Source: CAD feature listing. Evaluate the final solid. Frame: model axes, mm. Face numbers are marked on the shaded views. A direction names the side the tool comes from. Give positions to 0.01 mm unless a question says otherwise; leave off trailing zeros. Write each loop counter-clockwise with the first axis right and the second up, starting at its lowest first coordinate (ties: lowest second). Pieces come first, ordered by that corner, then holes. Notation, with made-up numbers: (18, 88.5) - (58, 88.5) arc R22 ccw to (58, 113.5) - close; hole circle Ø11 at (9, -25.5). An arc over 180 degrees is marked (long way). Answer as a JSON object with one key per item and string values. Group by question number.
from build123d import *

# Parameters (mm, degrees)
SKETCH1_R           = 2.794
BOSS_EXTRUDE1_DEPTH = 12.7
SKETCH2_R           = 1.778
CUT_EXTRUDE1_DEPTH  = 49.178879085
SKETCH4_R           = 4.953
CUT_EXTRUDE3_DEPTH  = 3.302
FILLET1_R           = 2.54
CUT_EXTRUDE4_DEPTH  = 3.302


with BuildPart() as part:
    # Sketch1 → Boss-Extrude1 (new body)
    with BuildSketch(Plane.XY):
        with BuildLine():
            ThreePointArc((28.575, 29.21), (27.831051224, 31.006051224), (26.035, 31.75))
            Line((26.035, 31.75), (16.32506331, 31.75))
            ThreePointArc((16.32506331, 31.75), (9.9441, 36.6522), (3.56313669, 31.75))
            Line((3.56313669, 31.75), (-3.56313669, 31.75))
            ThreePointArc((-3.56313669, 31.75), (-9.9441, 36.6522), (-16.32506331, 31.75))
            Line((-16.32506331, 31.75), (-26.035, 31.75))
            ThreePointArc((-26.035, 31.75), (-27.831051224, 31.006051224), (-28.575, 29.21))
            Line((-28.575, 29.21), (-28.575, -29.21))
            ThreePointArc((-28.575, -29.21), (-27.831051224, -31.006051224), (-26.035, -31.75))
            Line((-26.035, -31.75), (-16.32506331, -31.75))
            ThreePointArc((-16.32506331, -31.75), (-9.9441, -36.6522), (-3.56313669, -31.75))
            Line((-3.56313669, -31.75), (3.56313669, -31.75))
            ThreePointArc((3.56313669, -31.75), (9.9441, -36.6522), (16.32506331, -31.75))
            Line((16.32506331, -31.75), (26.035, -31.75))
            ThreePointArc((26.035, -31.75), (27.831051224, -31.006051224), (28.575, -29.21))
            Line((28.575, -29.21), (28.575, 29.21))
        make_face()
        with Locations((-9.9441, 30.0482)):
            Circle(SKETCH1_R, mode=Mode.SUBTRACT)
        with Locations((9.9441, 30.0482)):
            Circle(SKETCH1_R, mode=Mode.SUBTRACT)
        with Locations((9.9441, -30.0482)):
            Circle(SKETCH1_R, mode=Mode.SUBTRACT)
        with Locations((-9.9441, -30.0482)):
            Circle(SKETCH1_R, mode=Mode.SUBTRACT)
    extrude(amount=BOSS_EXTRUDE1_DEPTH)

    # Sketch2 → Cut-Extrude1 (cut, through all)
    with BuildSketch(Plane.XY.offset(12.7)):
        with Locations((-22.098, 19.3675)):
            Circle(SKETCH2_R)
        with Locations((-22.098, -12.5095)):
            Circle(SKETCH2_R)
        with Locations((22.606, -8.3693)):
            Circle(SKETCH2_R)
    extrude(amount=-CUT_EXTRUDE1_DEPTH, mode=Mode.SUBTRACT)

    # Sketch4 → Cut-Extrude3 (cut)
    with BuildSketch(Plane.XY.offset(12.7)):
        with Locations((-9.9441, 30.0482)):
            Circle(SKETCH4_R)
        with Locations((9.9441, 30.0482)):
            Circle(SKETCH4_R)
        with Locations((-9.9441, -30.0482)):
            Circle(SKETCH4_R)
        with Locations((9.9441, -30.0482)):
            Circle(SKETCH4_R)
    extrude(amount=-CUT_EXTRUDE3_DEPTH, mode=Mode.SUBTRACT)

    # Fillet1
    fillet1_edges = [part.edges().sort_by_distance(p)[0] for p in [
        (16.32506331, 31.75, 6.35),
        (16.32506331, -31.75, 6.35),
        (3.56313669, -31.75, 6.35),
        (-3.56313669, -31.75, 6.35),
        (-16.32506331, -31.75, 6.35),
        (-16.32506331, 31.75, 6.35),
        (-3.56313669, 31.75, 6.35),
        (3.56313669, 31.75, 6.35),
    ]]
    fillet(fillet1_edges, radius=FILLET1_R)

    # Sketch3 → Cut-Extrude4 (cut)
    with BuildSketch(Plane(origin=(0, 0, 0), x_dir=(-1, 0, 0), z_dir=(0, 0, -1))):
        Polygon((-22.606, -12.475415114), (-19.05, -10.422357557), (-19.05, -6.316242443), (-22.606, -4.263184886), (-26.162, -6.316242443), (-26.162, -10.422357557), align=None)
        Polygon((22.098, -16.615615114), (25.654, -14.562557557), (25.654, -10.456442443), (22.098, -8.403384886), (18.542, -10.456442443), (18.542, -14.562557557), align=None)
        Polygon((22.098, 15.261384886), (25.654, 17.314442443), (25.654, 21.420557557), (22.098, 23.473615114), (18.542, 21.420557557), (18.542, 17.314442443), align=None)
    extrude(amount=-CUT_EXTRUDE4_DEPTH, mode=Mode.SUBTRACT)


solid = part.part
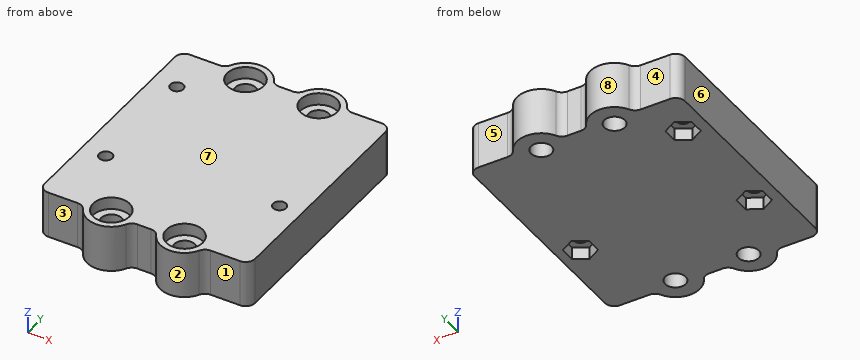
Q1. Draft query along X for the marked faces 6, 7 and 8. Return one class per face: released by +X, released by -X, zero draft, split by the parting line, or undercut.
Q2. Reachability of the marked faces 1, 2, 3, 4 and 5 from +Z, -Z, +X, -X, +Y, -Y: full face, straight path, thin tool, end or side. Return the list, or none.
Q3. First-contact query: pin 1 Ø6.5 at (x, z) = (22, 6.5) entering from -Y; pin 2 Ø4 at (x, z) = (18.5, 7) entering from -Y; pin 3 Ø1.5 at (x, z) = (-19.5, 7) entering from +Y. Flat tips, straight axial feed; report the tip coordinate or a pass-through.
Q4. Section C-C on x = -8.5. Return the cut outline in (y, z), then the cut area to 3 significant figures.
Q5. Ray query, probe 1 along Y at (x, z) = (12, 2.5); probe 2 along Y at (x, z) = (8, 4.25); probe 3 along X at (y, z) = (31, 9.25). Return the intervals inside material, ascending. Write a range as [from, to].
Q6. Section D-D on y = 16.5. Return the cut outline in (x, z) (3 decimals).
Q7. Section B-B on z = 5.75. State how many separate pieces and enclosed holes the cut face has, then the cut area to 3 significant figures.
Q8. Section A-A on x = 8. Return the cut outline in (y, z).
Taken from the geometry:
{
 "1": {"face 6": "released by -X", "face 7": "zero draft", "face 8": "undercut"},
 "2": {"face 1": "+Z, -Z, +X, -Y", "face 2": "+Z, -Z, -Y", "face 3": "+Z, -Z, -X, -Y", "face 4": "+Z, -Z, -X, +Y", "face 5": "+Z, -Z, +X, +Y"},
 "3": {"pin 1": "stops at y = -31.75", "pin 2": "stops at y = -32.27", "pin 3": "stops at y = 31.75"},
 "4": {"outline": "(-36.49, 0) - (-32.44, 0) - (-32.44, 9.4) - (-34.79, 9.4) - (-34.79, 12.7) - (-36.49, 12.7) - close; (-27.66, 0) - (27.66, 0) - (27.66, 9.4) - (25.31, 9.4) - (25.31, 12.7) - (-25.31, 12.7) - (-25.31, 9.4) - (-27.66, 9.4) - close; (32.44, 0) - (36.49, 0) - (36.49, 12.7) - (34.79, 12.7) - (34.79, 9.4) - (32.44, 9.4) - close", "area": "774 mm²"},
 "5": {"probe 1": "y = [-36.32, -31.94], [-28.16, 28.16], [31.94, 36.32]", "probe 2": "y = [-36.36, -32.05], [-28.04, 28.04], [32.05, 36.36]", "probe 3": "x = [-27.84, -12.57], [-7.32, 7.32], [12.57, 27.84]"},
 "6": {"outline": "(-28.575, 0) - (-24.243, 0) - (-24.243, 3.302) - (-19.953, 3.302) - (-19.953, 0) - (28.575, 0) - (28.575, 12.7) - (-28.575, 12.7) - close"},
 "7": {"separate pieces": "1", "enclosed holes": "7", "area": "3,680 mm²"},
 "8": {"outline": "(-36.36, 0) - (-32.05, 0) - (-32.05, 9.4) - (-34.6, 9.4) - (-34.6, 12.7) - (-36.36, 12.7) - close; (-28.04, 0) - (28.04, 0) - (28.04, 9.4) - (25.49, 9.4) - (25.49, 12.7) - (-25.49, 12.7) - (-25.49, 9.4) - (-28.04, 9.4) - close; (32.05, 0) - (36.36, 0) - (36.36, 12.7) - (34.6, 12.7) - (34.6, 9.4) - (32.05, 9.4) - close"}
}
